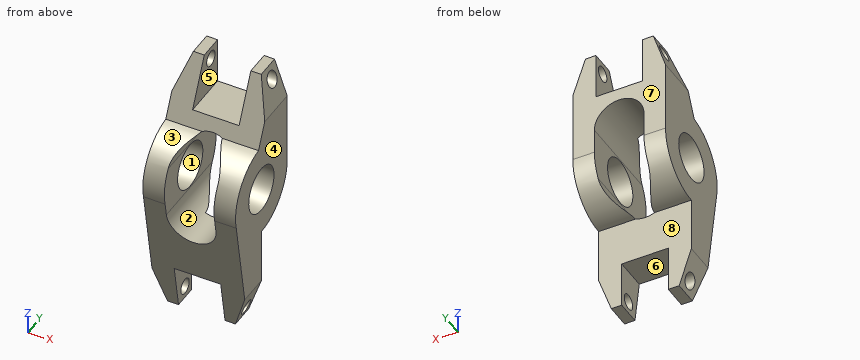
from build123d import *

# Parameters (mm, degrees)
SKETCH1_R               = 4.78
BOSS_EXTRUDE1_DEPTH     = 9.5
CUT_EXTRUDE1_DEPTH      = 32.661042702
CUT_EXTRUDE1_DEPTH_BACK = 32.661042702
SKETCH2_W               = 9.53
SKETCH2_H               = 9.53
CUT_EXTRUDE2_DEPTH      = 32.661042763
CUT_EXTRUDE2_DEPTH_BACK = 32.661042763
SKETCH3_R               = 1.59
CHAMFER1_SIZE           = 7.5
CHAMFER1_SIZE_2         = 2.6
CHAMFER2_SIZE           = 2.5
CHAMFER2_SIZE_2         = 7.6


with BuildPart() as part:
    # Sketch1 → Boss-Extrude1 (new, symmetric)
    with BuildSketch(Plane(origin=(0, 0, 0), x_dir=(0, 0, -1), z_dir=(1, 0, 0))):
        with BuildLine():
            Line((9.765, 0), (28.58, 0))
            Line((28.58, 0), (28.58, -5))
            Line((28.58, -5), (2.273512356, -9.496650281))
            ThreePointArc((2.273512356, -9.496650281), (-5.618124367, -7.986983385), (-9.706200338, -1.07))
            Line((-9.706200338, -1.07), (-22.23, 4.765))
            Line((-22.23, 4.765), (-22.23, 9.765))
            Line((-22.23, 9.765), (0, 9.765))
            ThreePointArc((0, 9.765), (6.904897718, 6.904897718), (9.765, 0))
        make_face()
        Circle(SKETCH1_R, mode=Mode.SUBTRACT)
    extrude(amount=BOSS_EXTRUDE1_DEPTH, both=True)

    # Sketch2 → Cut-Extrude1 (cut, two sides: drawn at the far end of the back side and taken through both)
    with BuildSketch(Plane(origin=(0, 0, 0), x_dir=(1, 0, 0), z_dir=(0, 1, 0)).offset(-CUT_EXTRUDE1_DEPTH_BACK)):
        with Locations((0, 23.815)):
            Rectangle(SKETCH2_W, SKETCH2_H)
        with BuildLine():
            Line((5.08, 5.08), (5.08, -5.08))
            ThreePointArc((5.08, -5.08), (0, -10.16), (-5.08, -5.08))
            Line((-5.08, -5.08), (-5.08, 5.08))
            ThreePointArc((-5.08, 5.08), (0, 10.16), (5.08, 5.08))
        make_face()
        with Locations((0, -17.465)):
            Rectangle(SKETCH2_W, SKETCH2_H)
    extrude(amount=CUT_EXTRUDE1_DEPTH + CUT_EXTRUDE1_DEPTH_BACK, mode=Mode.SUBTRACT)

    # Sketch3 → Cut-Extrude2 (cut, two sides: drawn at the far end of the back side and taken through both)
    with BuildSketch(Plane(origin=(0, 0, 0), x_dir=(0, 0, -1), z_dir=(1, 0, 0)).offset(-CUT_EXTRUDE2_DEPTH_BACK)):
        with Locations((-19.69, 7.225)):
            Circle(SKETCH3_R)
        with Locations((26.04, -2.54)):
            Circle(SKETCH3_R)
    extrude(amount=CUT_EXTRUDE2_DEPTH + CUT_EXTRUDE2_DEPTH_BACK, mode=Mode.SUBTRACT)

    # Chamfer1
    # the kernel refuses this chamfer: 7.5, 2.6 mm, written as the material it takes off along each edge
    with BuildSketch(Plane(origin=(9.5, -14.695177751, 22.23), x_dir=(0.01262359546550246, 0, -0.9999203192442502), z_dir=(0, 1, 0)), Plane(origin=(9.5, 19.460177751, -28.58), x_dir=(0.012623595465502456, 0, 0.9999203192442502), z_dir=(0, -1, 0))) as chamfer1_piece_1:
        Polygon((CHAMFER1_SIZE * 0.999920319244, CHAMFER1_SIZE * 0.0126235954655), (-CHAMFER1_SIZE_2 * 0.0126235954655, CHAMFER1_SIZE_2 * 0.999920319244), (0, 0), align=None)
    extrude(amount=43.920355501, mode=Mode.SUBTRACT)

    # Chamfer2
    # the kernel refuses this chamfer: 7.6, 2.5 mm, written as the material it takes off along each edge
    with BuildSketch(Plane(origin=(-9.5, -14.958373363, 22.23), x_dir=(0.9938650173465227, 0, 0.11059985214635677), z_dir=(0, 1, 0))) as chamfer2_piece_1:
        Polygon((CHAMFER2_SIZE * 0.993865017347, CHAMFER2_SIZE * 0.110599852146), (-CHAMFER2_SIZE_2 * 0.110599852146, CHAMFER2_SIZE_2 * 0.993865017347), (0, 0), align=None)
    extrude(amount=44.446746726, mode=Mode.SUBTRACT)
    with BuildSketch(Plane(origin=(-9.5, 19.723373363, -28.58), x_dir=(-0.012040610047615204, 0, 0.9999275092273846), z_dir=(0, -1, 0))) as chamfer2_piece_2:
        Polygon((CHAMFER2_SIZE_2 * 0.999927509227, -CHAMFER2_SIZE_2 * 0.0120406100476), (-CHAMFER2_SIZE * 0.0120406100476, -CHAMFER2_SIZE * 0.999927509227), (0, 0), align=None)
    extrude(amount=44.446746726, mode=Mode.SUBTRACT)


solid = part.part
Check sheet for the modelled part. Datum: model origin and axes. Units: mm. Face numbers are marked on the shaded views. A direction names the side the tool comes from. Give positions to 0.01 mm unless a question says otherwise; leave off trailing zeros. Write each loop counter-clockwise with the first axis right and the second up, starting at its lowest first coordinate (ties: lowest second). Pieces come first, ordered by that corner, then holes. Notation, with made-up numbers: (26.25, 28) -> (51.25, 28) arc R19 cw to (51.25, 53) -> close; hole circle Ø4 at (42.25, 15). An arc over 180 degrees is marked (long way). One line per item, written item: value. Start each with the question number.
Item 1: Section check A-A on y = -3.25. State how many separate pieces and enclosed holes the cut face has, then the cut area to 3 significant figures.
Item 2: Material ranges on probe 1 along Y at (x, z) = (-6.6, 0) (3 decimals); probe 2 along X at (y, z) = (-6, -5); probe 3 along Z at (x, y) = (3.75, -2), recorded low to high. Write a range as from..to.
Item 3: Section check B-B on z = 9. Record the cut outline in (x, y) (3 decimals), then the cut area to 3 significant figures.
Item 4: Tool access check on the marked faces 4, 5, 6, 7 and 8. Record the directions out of +Z, -Z, +X, -X, +Y, -Y that give a thin tool (end or side, any length) a straight path to the whole face; none if there is none.
Item 5: Section check C-C on z = 2. Record the cut outline in (x, y) (3 decimals).
Item 6: Draft check along Y on the marked faces 1, 2 and 3. Enter one of: +Y half, -Y half, draft (parallel to the pull), parting line (faces both ways), or undercut.
Item 7: Section check D-D on x = 0. Record the cut outline in (y, z) (3 decimals), then the cut area to 3 significant figures.
Item 8: Gauge pin test, flat ends, axial feed: pin 1 (4 mm diameter, centred on y = 7.225, z = 19.69, fed in from +X); pin 2 (3.5 mm diameter, centred on y = -4.5, z = -26, fed in from -X); pin 3 (3.5 mm diameter, centred on y = -3.5, z = -23.5, fed in from +X). Record the tip position at first contact, or that the pin passes through.
Results list:
1. separate pieces: 5
1. enclosed holes: 0
1. area: 348 mm²
2. probe 1: -9.765..-4.78, 4.78..9.765
2. probe 2: -9.5..-5.08, 5.08..9.5
2. probe 3: -19.05..-8.51, 8.51..9.56
3. outline: (-9.5, -3.789) -> (-3.231, -3.789) -> (-3.231, 9.765) -> (-9.5, 9.765) -> close; (3.231, -3.789) -> (9.5, -3.789) -> (9.5, 9.765) -> (3.231, 9.765) -> close
3. area: 170 mm²
4. face 4: +Z, -Z, +X, +Y, -Y
4. face 5: +Z, +Y, -Y
4. face 6: -Z, +Y, -Y
4. face 7: +Z, -Z, +X, -X, +Y
4. face 8: -Z, +X, -X, +Y
5. outline: (-9.5, -9.558) -> (-5.08, -9.558) -> (-5.08, -4.341) -> (-9.5, -4.341) -> close; (-9.5, 4.341) -> (-5.08, 4.341) -> (-5.08, 9.765) -> (-9.5, 9.765) -> close; (5.08, -9.558) -> (9.5, -9.558) -> (9.5, -4.341) -> (5.08, -4.341) -> close; (5.08, 4.341) -> (9.5, 4.341) -> (9.5, 9.765) -> (5.08, 9.765) -> close
6. face 1: undercut
6. face 2: draft
6. face 3: -Y half
7. outline: (-8.149, -10.16) -> (-6.629, -19.05) -> (0, -19.05) -> (0, -10.16) -> close; (-0.859, 10.16) -> (9.765, 10.16) -> (9.765, 12.7) -> (0.325, 12.7) -> close
7. area: 91.2 mm²
8. pin 1: x = 8.47
8. pin 2: x = -8.42
8. pin 3: x = 9.27
